Autodesk Inventor part; units mm, degrees
ref_plane "YZ Plane" through (0, 0, 0) normal (1, 0, 0) x (0, 1, 0)
ref_plane "XZ Plane" through (0, 0, 0) normal (0, 1, 0) x (-1, 0, 0)
ref_plane "XY Plane" through (0, 0, 0) normal (0, 0, 1) x (1, 0, 0)
sketch "Sketch2" plane through (0, 0, 0) normal (0, 0, 1) x (1, 0, 0)
  line L0 (-10.25, -25) -> (-6.25, -25)
  line L1 (-3.25, -22) -> (-3.25, 13)
  line L2 (-0.25, 16) -> (0.25, 16)
  line L3 (3.25, 13) -> (3.25, -22)
  line L4 (6.25, -25) -> (10.25, -25)
  line L5 (29.5, 46) -> (-29.5, 46)
  line L6 (-32.5, 43) -> (-32.5, 9)
  line L7 (0, 0) -> (0, 46) construction
  circle A0 centre (-17.5, 38) radius 1.6
  circle A1 centre (17.5, 38) radius 1.6
  circle A2 centre (-8.05, -20) radius 1.6
  circle A3 centre (8.05, -20) radius 1.6
  line L8 (0, 0) -> (32.5, 0) construction
  arc A4 (-0.25, 16) -> (-3.25, 13) centre (-0.25, 13) ccw
  arc A5 (3.25, 13) -> (0.25, 16) centre (0.25, 13) ccw
  arc A6 (-29.5, 46) -> (-32.5, 43) centre (-29.5, 43) ccw
  arc A7 (32.5, 43) -> (29.5, 46) centre (29.5, 43) ccw
  arc A8 (3.25, -22) -> (6.25, -25) centre (6.25, -22) ccw
  arc A9 (-6.25, -25) -> (-3.25, -22) centre (-6.25, -22) ccw
  circle A10 centre (-27.5, 13) radius 1.3
  line L9 (29.5, 6) -> (16.25, 6)
  line L10 (13.25, 3) -> (13.25, -22)
  line L11 (-29.5, 6) -> (-16.25, 6)
  line L12 (-13.25, 3) -> (-13.25, -22)
  line L13 (32.5, 9) -> (32.5, 43)
  arc A11 (10.25, -25) -> (13.25, -22) centre (10.25, -22) ccw
  arc A12 (-13.25, -22) -> (-10.25, -25) centre (-10.25, -22) ccw
  arc A13 (16.25, 6) -> (13.25, 3) centre (16.25, 3) ccw
  arc A14 (-13.25, 3) -> (-16.25, 6) centre (-16.25, 3) ccw
  arc A15 (29.5, 6) -> (32.5, 9) centre (29.5, 9) ccw
  arc A16 (-32.5, 9) -> (-29.5, 6) centre (-29.5, 9) ccw
  point P0 (-3.25, 16)
  point P1 (3.25, 16)
  point P2 (3.25, -25)
  point P3 (32.5, 6)
  point P4 (13.25, 6)
  point P5 (-13.25, 6)
  point P6 (13.25, -25)
  point P7 (-13.25, -25)
  point P8 (-32.5, 6)
  dimension "d1" = 16.1
  dimension "d3" = 16
  dimension "d4" = 20
  dimension "d5" = 5
  dimension "d6" = 6.5
  dimension "d7" = 3.2
  dimension "d13" = 8
  dimension "d14" = 15
  dimension "d16" = 30
  dimension "d18" = 3.2
  dimension "d19" = 3
  dimension "d20" = 3
  dimension "d23" = 5
  dimension "d24" = 33
  dimension "d25" = 2.6
  dimension "d26" = 32.5
  dimension "d27" = 10
  dimension "d28" = 3
  dimension "d29" = 40
extrude "Extrusion1" add sketch "Sketch2" along normal blind 3.175
sketch "Sketch3" plane through (0, 0, 0) normal (0, 0, -1) x (-1, 0, 0)
  circle A0 centre (0, 26) radius 3.4
  circle A1 centre (18, 26) radius 3.4
  circle A2 centre (-18, 26) radius 3.4
  line L0 (-29.5, 46) -> (29.5, 46)
  line L1 (-32.5, 9) -> (-32.5, 43) construction
  line L2 (-32.5, 26) -> (32.5, 26) construction
  line L3 (32.5, 43) -> (32.5, 9) construction
  line L4 (-18, 26) -> (18, 26) construction
  line L5 (-29.5, 46) -> (29.5, 46) construction
  line L6 (0, 46) -> (0, 26) construction
  circle A3 centre (-26, 19.5) radius 1
  circle A4 centre (26, 19.5) radius 1
  line L7 (0, 26) -> (0, 46) construction
  point P0 (0, 0)
  dimension "d30" = 6.8
  dimension "d34" = 18
  dimension "d35" = 18
  dimension "d38" = 52
  dimension "d39" = 6.5
  dimension "d40" = 2
extrude "Extrusion2" cut sketch "Sketch3" against normal up to next
properties part number "shovel_mount"
Input: part model. Units: mm. Frame: model coordinates. A direction names the side the tool comes from. Round coordinates to 2 decimals unless told otherwise and drop trailing zeros. Order: outer loops, then holes, each group sorted by start corner. A loop starts at its lowest first (then second) coordinate and runs counter-clockwise, first axis right, second up. Notation, with made-up numbers: (89, -19) - (118, -19) arc R14 cw to (118, -5) - close; hole circle Ø3 at (61.25, -25.75). An arc over 180 degrees is marked (long way). Answer in a Markdown table with one row per item.
Item 1: Reachability of faces 4 (the cylindrical face through (4.15, -24.14, 1.57)), 5 (the flat face through (13.25, -9, 2)), 6 (the flat face through (-32.5, 26, 2)), 7 (the cylindrical face through (-28.8, 12.94, 1.57)), 8 (the flat face through (-23, 6, 2)) from +Z, -Z, +X, -X, +Y, -Y: full face, straight path, thin tool, end or side. Return the list, or none.
Model answer:
| item | result |
|---|---|
| face 4 | +Z, -Z, -Y |
| face 5 | +Z, -Z, +X, -Y |
| face 6 | +Z, -Z, -X, +Y, -Y |
| face 7 | +Z, -Z |
| face 8 | +Z, -Z, -X, -Y |
Item 2: Pin query (flat end, axial travel): pin 1 (1 mm diameter, centred on y = -12, z = 2, fed in from +X); pin 2 (3 mm diameter, centred on x = 17.5, y = 38, fed in from +Z); pin 3 (1 mm diameter, centred on y = -10, z = 1.5, fed in from -X); pin 4 (1.6 mm diameter, centred on x = 25, z = 1, fed in from -Y). Return the tip coordinate at first contact, or that it passes through.
Model answer:
| item | result |
|---|---|
| pin 1 | stops at x = 13.25 |
| pin 2 | passes through |
| pin 3 | stops at x = -13.25 |
| pin 4 | stops at y = 6 |
Item 3: Section query B-B (z = 0.85). Give the number of separate pieces and of enclosed holes in the cut face, then the cut area to 3 significant figures.
Model answer:
| item | result |
|---|---|
| separate pieces | 1 |
| enclosed holes | 10 |
| area | 2,990 mm² |
Item 4: Section query C-C (y = -2.5). Return the cut outline in (x, z) (3 decimals).
Model answer:
| item | result |
|---|---|
| outline | (-13.25, 0) - (-3.25, 0) - (-3.25, 3.175) - (-13.25, 3.175) - close; (3.25, 0) - (13.25, 0) - (13.25, 3.175) - (3.25, 3.175) - close |
Item 5: Section query D-D (y = -20). Return the cut outline in (x, z) (3 decimals), then the cut area to 3 significant figures.
Model answer:
| item | result |
|---|---|
| outline | (-13.25, 0) - (-9.65, 0) - (-9.65, 3.175) - (-13.25, 3.175) - close; (-6.45, 0) - (-3.25, 0) - (-3.25, 3.175) - (-6.45, 3.175) - close; (3.25, 0) - (6.45, 0) - (6.45, 3.175) - (3.25, 3.175) - close; (9.65, 0) - (13.25, 0) - (13.25, 3.175) - (9.65, 3.175) - close |
| area | 43.2 mm² |
Item 6: Mould query, pull axis Y, two halves, no side actions, for faces 1 (the cylindrical face through (-25.783, 18.524, 1.565)), 2 (the cylindrical face through (31.64, 6.9, 1.57)), 3 (the flat face through (-3.25, -5, 2)). Classes: released by +Y, released by -Y, zero draft, split by the parting line, or undercut.
Model answer:
| item | result |
|---|---|
| face 1 | undercut |
| face 2 | released by -Y |
| face 3 | zero draft |
Item 7: Section query A-A (y = 38). Return the cut outline in (x, z) (3 decimals).
Model answer:
| item | result |
|---|---|
| outline | (-32.5, 0) - (-19.1, 0) - (-19.1, 3.175) - (-32.5, 3.175) - close; (-15.9, 0) - (15.9, 0) - (15.9, 3.175) - (-15.9, 3.175) - close; (19.1, 0) - (32.5, 0) - (32.5, 3.175) - (19.1, 3.175) - close |
Item 8: Line query: line 1 (X direction, y = -18, z = 2.6); line 2 (Y direction, x = 18, z = 0.75); line 3 (Y direction, x = 0, z = 2). Output: solid intervals per line, ascending.
Model answer:
| item | result |
|---|---|
| line 1 | x = -13.25 to -3.25, 3.25 to 13.25 |
| line 2 | y = 6 to 22.6, 29.4 to 36.48, 39.52 to 46 |
| line 3 | y = 16 to 22.6, 29.4 to 46 |
